Autodesk Inventor part; units mm, degrees
ref_plane "YZ Plane" through (0, 0, 0) normal (1, 0, 0) x (0, 1, 0)
ref_plane "XZ Plane" through (0, 0, 0) normal (0, 1, 0) x (-1, 0, 0)
ref_plane "XY Plane" through (0, 0, 0) normal (0, 0, 1) x (1, 0, 0)
sketch "Sketch1" plane through (0, 0, 0) normal (0, 0, 1) x (1, 0, 0)
  line L0 (0, 0) -> (252.4125, 0)
  line L1 (252.4125, 0) -> (252.4125, 244.475)
  line L2 (252.4125, 244.475) -> (0, 244.475)
  line L3 (0, 244.475) -> (0, 0)
  dimension "d0" = 252.4125
  dimension "d1" = 244.475
extrude "Extrusion1" add sketch "Sketch1" along normal blind 19.05
sketch "Sketch3" plane through (0, 0, 19.05) normal (0, 0, 1) x (1, 0, 0)
  line L0 (0, 0) -> (252.4125, 0)
  line L1 (252.4125, 244.475) -> (0, 244.475)
  line L2 (0, 244.475) -> (0, 0)
  line L3 (0, 244.475) -> (19.05, 244.475)
  line L4 (19.05, 244.475) -> (19.05, 225.425)
  line L5 (19.05, 225.425) -> (0, 225.425)
  line L6 (0, 225.425) -> (0, 244.475)
  line L7 (19.05, 168.275) -> (0, 168.275)
  line L8 (0, 168.275) -> (0, 149.225)
  line L9 (0, 149.225) -> (19.05, 149.225)
  line L10 (19.05, 149.225) -> (19.05, 168.275)
  line L11 (0, 130.175) -> (19.05, 130.175)
  line L12 (19.05, 130.175) -> (19.05, 111.125)
  line L13 (19.05, 111.125) -> (0, 111.125)
  line L14 (0, 111.125) -> (0, 130.175)
  line L15 (0, 206.375) -> (19.05, 206.375)
  line L16 (19.05, 206.375) -> (19.05, 187.325)
  line L17 (19.05, 187.325) -> (0, 187.325)
  line L18 (0, 187.325) -> (0, 206.375)
  line L19 (0, 92.075) -> (19.05, 92.075)
  line L20 (19.05, 92.075) -> (19.05, 73.025)
  line L21 (19.05, 73.025) -> (0, 73.025)
  line L22 (0, 73.025) -> (0, 92.075)
  line L23 (0, 53.975) -> (19.05, 53.975)
  line L24 (19.05, 53.975) -> (19.05, 34.925)
  line L25 (19.05, 34.925) -> (0, 34.925)
  line L26 (0, 34.925) -> (0, 53.975)
  line L27 (0, 15.875) -> (19.05, 15.875)
  line L28 (19.05, 15.875) -> (19.05, -3.175)
  line L29 (19.05, -3.175) -> (0, -3.175)
  line L30 (0, -3.175) -> (0, 15.875)
  dimension "d4" = 19.05
  dimension "d5" = 19.05
  dimension "d6" = 244.475
  dimension "d7" = 19.05
  dimension "d8" = 19.05
  dimension "d9" = 19.05
  dimension "d10" = 19.05
  dimension "d11" = 19.05
  dimension "d12" = 19.05
  dimension "d13" = 19.05
  dimension "d14" = 19.05
  dimension "d15" = 19.05
  dimension "d16" = 19.05
  dimension "d17" = 19.05
  dimension "d18" = 19.05
  dimension "d19" = 19.05
  dimension "d20" = 19.05
  dimension "d21" = 19.05
  dimension "d22" = 19.05
  dimension "d23" = 19.05
  dimension "d24" = 15.875
extrude "Extrusion2" cut sketch "Sketch3" against normal through all
mirror "Mirror1" about plane through (252.4125, 0, 0) normal (1, 0, 0)
properties part number "deep_side" material "Wood (Birch)"
Can you work these out from the model? Positions are in its coordinate system, mm. A direction names the side the tool comes from. Coordinates: 2 decimals unless noted, no trailing zeros. Write each loop counter-clockwise with the first axis right and the second up, starting at its lowest first coordinate (ties: lowest second). Pieces come first, ordered by that corner, then holes. Notation, with made-up numbers: (81.5, 7) -> (129.5, 7) arc R17 cw to (129.5, 38) -> close; hole circle Ø8 at (47.25, 76). An arc over 180 degrees is marked (long way). Write each question's results on one line, items separated by ' | '. Start each with the question number.
Q1. If I drill on probe 1 along X at (y, z) = (165.5, 16) (3 decimals), over which ranges is the centre line in solid material (lowest first)?
Q2. On a 3-axis mill with a long thin cutter (end or side, diameter ignored), from which of +Z, -Z, +X, -X, +Y, -Y can I reach the whole of each face in a straight line? I mean faces 1 (the face through (495, 53.975, 10)), 2 (the face through (19.05, 8, 10)), 3 (the face through (485.775, 235, 10)), 4 (the face through (19.05, 197, 10)). Say none if no direction works.
Q3. Imagine slicing it at A-A (y = 83.5). Write out the boundary of the cut face in (x, z) (3 decimals).
Q4. I'm going to push flat-ended pins straight in: pin 1 (6 mm diameter, centred on y = 116.5, z = 16, fed in from -X); pin 2 (9.5 mm diameter, centred on x = 10, z = 8, fed in from -Y) (3 decimals); pin 3 (5.5 mm diameter, centred on x = 500, z = 6.5, fed in from +Y) (3 decimals). Where does each tip first touch, or does it pass through?
Q5. We'd pull the mould along Y, two halves only. Please class faces 5 (the face through (495, 225.425, 10)), 6 (the face through (19.05, 235, 10)), 7 (the face through (10, 111.125, 10)): +Y half, -Y half, draft (parallel to the pull), parting line (faces both ways), or undercut.
Taken from the geometry:
1) probe 1: x = 19.05 to 485.775
2) face 1: +Z, -Z, +X | face 2: +Z, -Z, -X, -Y | face 3: +Z, -Z, +X, +Y | face 4: +Z, -Z, -X
3) outline: (19.05, 0) -> (485.775, 0) -> (485.775, 19.05) -> (19.05, 19.05) -> close
4) pin 1: stops at x = 19.05 | pin 2: stops at y = 15.875 | pin 3: stops at y = 225.425
5) face 5: +Y half | face 6: draft | face 7: undercut
